Autodesk Inventor part; units mm, degrees
ref_plane "Konstruktionshilfsebene" through (25, 30, 0) normal (-1, 0, 0) x (0, -1, 0)
ref_plane "YZ Plane" through (0, 0, 0) normal (1, 0, 0) x (0, 1, 0)
ref_plane "XZ Plane" through (0, 0, 0) normal (0, 1, 0) x (-1, 0, 0)
sketch "Skizze1" plane through (0, 0, 0) normal (0, 0, 1) x (1, 0, 0)
  line L0 (0, 0) -> (55, 0)
  line L1 (55, 0) -> (55, 60)
  line L2 (55, 60) -> (0, 60)
  line L3 (0, 60) -> (0, 0)
  dimension "d0" = 60
  dimension "d1" = 55
extrude "Grundkörper" add sketch "Skizze1" along normal blind 40
fillet "Konturverrundung" radius 30 2 edges at (55, 60, 20) (55, 0, 20)
sketch "Skizze2" plane through (0, 0, 40) normal (0, 0, 1) x (1, 0, 0)
  point P0 (0, 0)
  point P1 (25, 30)
  point P2 (25, 30)
hole "Durchgangsbohrung 60H7" at (25, 30, 40) direction (0, 0, -1) diameter 55 end through all
sketch "Skizze3" plane through (0, 0, 0) normal (-1, 0, 0) x (0, 0, 1)
  line L0 (0, 0) -> (40, 0) construction
  line L1 (40, 60) -> (40, 0) construction
  line L2 (0, 0) -> (40, 60) construction
  line L3 (0, 60) -> (40, 60) construction
  line L4 (0, 60) -> (40, 0) construction
  line L5 (0, 85) -> (40, 85)
  line L6 (40, 85) -> (40, -25)
  line L7 (40, -25) -> (0, -25)
  line L8 (0, -25) -> (0, 85)
  line L9 (0, 85) -> (40, -25) construction
  line L10 (40, 85) -> (0, -25) construction
  point P0 (20, 30)
  dimension "d16" = 110
extrude "Aufnahmeplatte" add sketch "Skizze3" along normal blind 15
sketch "Skizze4" plane through (0, 0, 0) normal (1, 0, 0) x (0, 0, -1)
  line L0 (-40, 85) -> (0, 85)
  line L1 (-20, 85) -> (-20, -25)
  line L2 (-40, -25) -> (0, -25)
  line L3 (0, 60) -> (-40, 60)
  line L4 (8, 30) -> (-48, 30)
  point P0 (0, 0)
  point P1 (-20, 72.5)
  point P2 (-20, -12.5)
  dimension "d26" = 25
  dimension "d27" = 12.5
hole "Senkung_Zylinderkopfschraube M6" at (0, 72.5, 20) at (0, -12.5, 20) direction (-1, 0, 0) diameter 6.6 end through all counterbore diameter 11 counterbore depth 6.6
ref_plane "Konstruktionshilfsebene" through (25, 30, 0) normal (-1, 0, 0) x (0, -1, 0)
ref_plane "Arbeitsebene3" through (55, 30, 0) normal (-1, 0, 0) x (0, -1, 0)
sketch "Skizze6" plane through (25, 30, 0) normal (-1, 0, 0) x (0, -1, 0)
  line L0 (-27.5, 0) -> (-27.5, 40) construction
  line L1 (-6.1835, 0) -> (-3.8165, 0) construction
  line L2 (0, 0) -> (0, 40) construction
  line L3 (-27.5, 40) -> (27.5, 40) construction
  line L4 (-27.5, 40) -> (-23.5, 40)
  line L5 (-23.5, 40) -> (-23.5, 28.5)
  line L6 (-23.5, 28.5) -> (-20, 28.5)
  line L7 (-20, 28.5) -> (-20, 24)
  line L8 (-17.5, 24) -> (-17.5, 19)
  line L9 (-17.5, 19) -> (-21, 19)
  line L10 (-21, 19) -> (-21, 7)
  line L11 (-21, 7) -> (-21, 7)
  line L12 (-22, 6) -> (-22, 0)
  line L13 (27.5, 0) -> (-27.5, 0) construction
  line L14 (-22, 0) -> (-27.5, 0)
  line L15 (-21, 7) -> (-22, 6)
  line L16 (-27.5, 40) -> (-27.5, 0)
  line L17 (-20, 24) -> (-17.5, 24)
  point P0 (30, 0)
  point P1 (-22, 7)
  dimension "d46" = 47
  dimension "d47" = 11.5
  dimension "d48" = 40
  dimension "d49" = 35
  dimension "d52" = 33
  dimension "d53" = 21
  dimension "d54" = 42
  dimension "d55" = 44
  dimension "d57" = 1
  dimension "d58" = 1
  dimension "d79" = 9.5
  dimension "d80" = 16
revolve "Lagersitz" add sketch "Skizze6" angle 360 about axis through (25, 30, 0) along (0, 0, 1)
sketch "Skizze8" plane through (0, 0, 0) normal (0, 0, -1) x (-1, 0, 0)
  circle A0 centre (-25, 30) radius 17.5 construction
  line L0 (-25, 60) -> (0, 60) construction
  line L1 (-25, 30) -> (-25, 60) construction
  line L2 (-25, 30) -> (-55, 30) construction
  arc A1 (-25, 60) -> (-25, 0) centre (-25, 30) ccw construction
  circle A2 centre (-25, 30) radius 26 construction
  point P0 (0, 0)
  point P1 (-25, 56)
  point P2 (-51, 30)
  point P3 (-25, 4)
  point P4 (1, 30)
  dimension "d68" = 52
  dimension "d67" = 30
  dimension "d71" = 360
hole "Gewinde_Keine_ISO Metrisches Profil_2_Winkel(5)" at (25, 56, 0) at (51, 30, 0) at (25, 4, 0) at (-1, 30, 0) direction (0, 0, 1) diameter 1.567 depth 10 tip angle 118
chamfer "Gewindesenkung 0.4mm" distance 0.4 angle 45 4 edges at (25, 55.2165, 0) (51, 29.2165, 0) (-1, 29.2165, 0) (25, 3.2165, 0)
chamfer "Fase4" distance 0.5 angle 45 1 edges at (25, 6.5, 40)
properties part number "shoulder_joint_fit_v2" material "Stahl, hochfest, niedrig legiert"
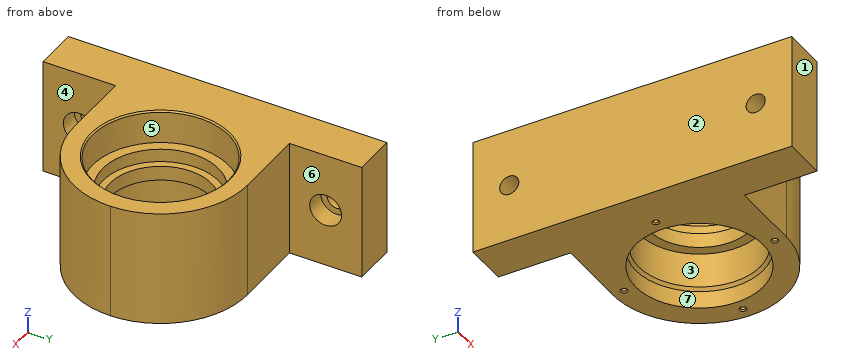
Work out the finished part from the listing and answer in its coordinate system (mm). Face numbers are marked on the shaded views. A direction names the side the tool comes from. Give positions to 0.01 mm unless a question says otherwise; leave off trailing zeros. Order: outer loops, then holes, each group sorted by start corner. A loop starts at its lowest first (then second) coordinate and runs counter-clockwise, first axis right, second up.
1. Each of these flat-tipped pins is pushed along its axis until it touches: P1, Ø12.5, axis at y = -15, z = 29.5, coming from the +X side; P2, Ø4, axis at x = 39, z = 20.5, coming from the +Y side; P3, Ø10.5, axis at y = 72.5, z = 20, coming from the +X side. Where does it stop, or does it pass through?
Result sheet:
P1: stops at x = 0
P2: stops at y = 57.5
P3: stops at x = -6.6
2. Straight lines are drawn through the part: L1, parallel to X at y = 30, z = 2.5; L2, parallel to Z at x = -2.25, y = -12.5; L3, parallel to Y at x = 25, z = 2.75. For each, find the intervals that lie inside material, in ascending order.
Result sheet:
L1: x = -15 to -1.78, -0.22 to 3, 47 to 50.22, 51.78 to 55
L2: z = 0 to 14.5, 25.5 to 40
L3: y = 0 to 3.22, 4.78 to 8, 52 to 55.22, 56.78 to 60
3. Section A-A, the plane y = 1.5 is taken. Determine the outline of the cut face in (x, z), and give its area (3 significant figures).
Result sheet:
outline: (-15, 0) - (34.37, 0) - (34.37, 40) - (-15, 40) - close
area: 1,970 mm2
4. For the marked faces 4, 5, 6 and 7, determine the directions among +Z, -Z, +X, -X, +Y, -Y from which every point of the face is accessible in a straight line to the end or side of a thin tool.
Result sheet:
face 4: +Z, -Z, +X, -Y
face 5: +Z
face 6: +Z, -Z, +X, +Y
face 7: -Z
5. The mould has two halves that part along Y. Classify the marked faces 1, 2 and 3: released by +Y, released by -Y, zero draft, split by the parting line, or undercut.
Result sheet:
face 1: released by -Y
face 2: zero draft
face 3: undercut
